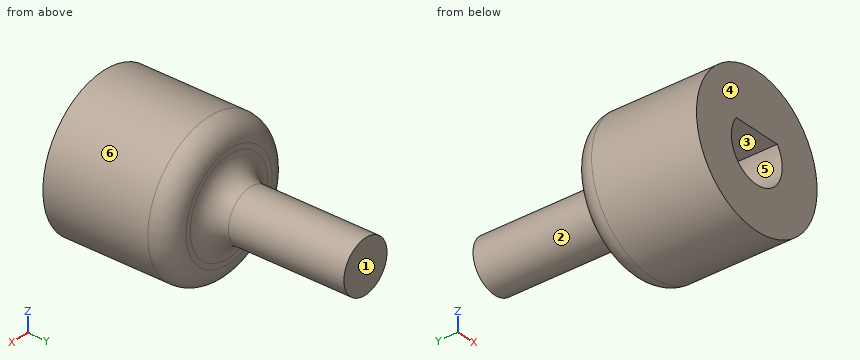
from build123d import *

# Parameters (mm, degrees)
SKETCH1_R           = 12.5
SKETCH1_R_2         = 2
BOSS_EXTRUDE1_DEPTH = 5
SKETCH2_R           = 2.5
BOSS_EXTRUDE2_DEPTH = 15
SKETCH3_R           = 5
CUT_EXTRUDE1_DEPTH  = 2
SKETCH4_R           = 12.5
CUT_EXTRUDE2_DEPTH  = 24.184046239
SKETCH5_R           = 7
SKETCH5_R_2         = 2.95
BOSS_EXTRUDE3_DEPTH = 10
SKETCH5_3_R         = 7
SKETCH5_3_R_2       = 2.95
BOSS_EXTRUDE4_DEPTH = 2
FILLET1_R           = 2
FILLET2_R           = 2


with BuildPart() as part:
    # Sketch1 → Boss-Extrude1 (new body)
    with BuildSketch(Plane(origin=(0, 0, 0), x_dir=(1, 0, 0), z_dir=(0, 1, 0))):
        with Locations(Location((0, 0, 0), (0, 0, 270))):
            Circle(SKETCH1_R)
        with Locations(Location((-7.5, 0, 0), (0, 0, 270))):
            Circle(SKETCH1_R_2, mode=Mode.SUBTRACT)
        with Locations(Location((0, 7.5, 0), (0, 0, 270))):
            Circle(SKETCH1_R_2, mode=Mode.SUBTRACT)
        with Locations(Location((7.5, 0, 0), (0, 0, 270))):
            Circle(SKETCH1_R_2, mode=Mode.SUBTRACT)
        with Locations(Location((0, -7.5, 0), (0, 0, 270))):
            Circle(SKETCH1_R_2, mode=Mode.SUBTRACT)
    extrude(amount=BOSS_EXTRUDE1_DEPTH)

    # Sketch2 → Boss-Extrude2 (add)
    with BuildSketch(Plane(origin=(0, 5, 0), x_dir=(1, 0, 0), z_dir=(0, 1, 0))):
        with Locations(Location((0, 0, 0), (0, 0, 270))):
            Circle(SKETCH2_R)
    extrude(amount=BOSS_EXTRUDE2_DEPTH)

    # Sketch3 → Cut-Extrude1 (cut)
    with BuildSketch(Plane.XZ):
        with Locations(Location((0, 0, 0), (0, 0, 270))):
            Circle(SKETCH3_R)
    extrude(amount=-CUT_EXTRUDE1_DEPTH, mode=Mode.SUBTRACT)

    # Sketch4 → Cut-Extrude2 (cut, through all)
    with BuildSketch(Plane(origin=(0, 5, 0), x_dir=(1, 0, 0), z_dir=(0, 1, 0))):
        Circle(SKETCH4_R)
    extrude(amount=-CUT_EXTRUDE2_DEPTH, mode=Mode.SUBTRACT)

    # Sketch5 → Boss-Extrude3 (add)
    with BuildSketch(Plane.XZ.offset(-5)):
        with Locations(Location((0, 0, 0), (0, 0, 270))):
            Circle(SKETCH5_R)
        Circle(SKETCH5_R_2, mode=Mode.SUBTRACT)
        with BuildLine():
            Line((-1.785357107, 1.75), (0, 1.75))
            Line((0, 1.75), (1.785357107, 1.75))
            ThreePointArc((1.785357107, 1.75), (0, 2.5), (-1.785357107, 1.75))
        make_face()
        with BuildLine():
            ThreePointArc((2.374868417, 1.75), (0, 2.95), (-2.374868417, 1.75))
            Line((-2.374868417, 1.75), (-1.785357107, 1.75))
            ThreePointArc((-1.785357107, 1.75), (0, 2.5), (1.785357107, 1.75))
            Line((1.785357107, 1.75), (2.374868417, 1.75))
        make_face()
    extrude(amount=BOSS_EXTRUDE3_DEPTH)

    # Sketch5_3 → Boss-Extrude4 (add)
    with BuildSketch(Plane.XZ.offset(-5)):
        with Locations(Location((0, 0, 0), (0, 0, 270))):
            Circle(SKETCH5_3_R)
        Circle(SKETCH5_3_R_2, mode=Mode.SUBTRACT)
        with BuildLine():
            Line((-1.785357107, 1.75), (0, 1.75))
            Line((0, 1.75), (1.785357107, 1.75))
            ThreePointArc((1.785357107, 1.75), (0, 2.5), (-1.785357107, 1.75))
        make_face()
        with BuildLine():
            ThreePointArc((2.374868417, 1.75), (0, 2.95), (-2.374868417, 1.75))
            Line((-2.374868417, 1.75), (-1.785357107, 1.75))
            ThreePointArc((-1.785357107, 1.75), (0, 2.5), (1.785357107, 1.75))
            Line((1.785357107, 1.75), (2.374868417, 1.75))
        make_face()
        with BuildLine():
            ThreePointArc((-2.374868417, 1.75), (-2.632964109, -1.33041347), (0, -2.95))
            Line((0, -2.95), (0, -2.5))
            ThreePointArc((0, -2.5), (-2.304886114, -0.968245837), (-1.785357107, 1.75))
            Line((-1.785357107, 1.75), (-2.374868417, 1.75))
        make_face()
        with BuildLine():
            Line((0, -2.5), (0, -2.95))
            ThreePointArc((0, -2.95), (2.085965005, -2.085965005), (2.95, 0))
            ThreePointArc((2.95, 0), (2.802531162, 0.92104239), (2.374868417, 1.75))
            Line((2.374868417, 1.75), (1.785357107, 1.75))
            ThreePointArc((1.785357107, 1.75), (2.314453798, 0.945147404), (2.5, 0))
            ThreePointArc((2.5, 0), (1.767766953, -1.767766953), (0, -2.5))
        make_face()
        with BuildLine():
            ThreePointArc((-1.785357107, 1.75), (-2.304886114, -0.968245837), (0, -2.5))
            Line((0, -2.5), (0, 1.75))
            Line((0, 1.75), (-1.785357107, 1.75))
        make_face()
        with BuildLine():
            Line((0, 1.75), (0, -2.5))
            ThreePointArc((0, -2.5), (1.767766953, -1.767766953), (2.5, 0))
            ThreePointArc((2.5, 0), (2.314453798, 0.945147404), (1.785357107, 1.75))
            Line((1.785357107, 1.75), (0, 1.75))
        make_face()
    extrude(amount=-BOSS_EXTRUDE4_DEPTH)

    # Fillet1
    fillet1_edges = [part.edges().sort_by_distance(p)[0] for p in [
        (0, 7, -2.5),
    ]]
    fillet(fillet1_edges, radius=FILLET1_R)

    # Fillet2
    fillet2_edges = [part.edges().sort_by_distance(p)[0] for p in [
        (0, 7, 7),
    ]]
    fillet(fillet2_edges, radius=FILLET2_R)


solid = part.part
Part model, mm, in its own coordinate system. Face numbers are marked on the shaded views. A direction names the side the tool comes from. Coordinates: 2 decimals unless noted, no trailing zeros. Write each loop counter-clockwise with the first axis right and the second up, starting at its lowest first coordinate (ties: lowest second). Pieces come first, ordered by that corner, then holes. Notation, with made-up numbers: (60.25, 29.5) - (70.25, 29.5) arc R30 ccw to (70.25, 61.5) - close; hole circle Ø4 at (44.25, 89.5). An arc over 180 degrees is marked (long way). Put each result on its own line as item: value.
1. 3-axis set-ups, long thin cutter, end or side, ignore diameter. For the marked faces 1 and 2: which of +Z, -Z, +X, -X, +Y, -Y reach the whole face in a straight line?
Final values:
face 1: +Z, -Z, +X, -X, +Y
face 2: +Y
2. Probe line 1 along X through (y, z) = (1.75, 0); line 2 along X through (y, z) = (-1, 1); line 3 along Z through (x, y) = (2.5, 2.75). List the from-to ranges inside material, lowest first. Write a range as [from, to].
Final values:
line 1: x = [-7, -2.95], [2.95, 7]
line 2: x = [-6.93, -2.78], [2.78, 6.93]
line 3: z = [-6.54, -1.57], [1.57, 6.54]
3. Band-saw the part on A-A (x = 0). Write the cut outline in (y, z).
Final values:
outline: (-5, -7) - (5, -7) arc R2 ccw to (7, -5) - (7, -4.5) arc R2 cw to (9, -2.5) - (20, -2.5) - (20, 2.5) - (9, 2.5) arc R2 cw to (7, 4.5) - (7, 5) arc R2 ccw to (5, 7) - (-5, 7) - (-5, 1.75) - (5, 1.75) - (5, -2.95) - (-5, -2.95) - close
4. Band-saw the part on B-B (z = 0). Write the cut outline in (x, y).
Final values:
outline: (-7, -5) - (-2.95, -5) - (-2.95, 5) - (2.95, 5) - (2.95, -5) - (7, -5) - (7, 5) arc R2 ccw to (5, 7) - (4.5, 7) arc R2 cw to (2.5, 9) - (2.5, 20) - (-2.5, 20) - (-2.5, 9) arc R2 cw to (-4.5, 7) - (-5, 7) arc R2 ccw to (-7, 5) - close
5. Band-saw the part on C-C (y = -1.25). Write the cut outline in (x, z).
Final values:
outline: circle Ø14 at (0, 0); hole (-2.37, 1.75) arc R2.95 ccw (long way) to (2.37, 1.75) - close
6. Band-saw the part on D-D (y = 17). Write the cut outline in (x, z).
Final values:
outline: circle Ø5 at (0, 0)
7. Two-plate mould, pull along Z, no slides. Class the marked faces 3, 4, 5 and 6: +Z half, -Z half, draft (parallel to the pull), parting line (faces both ways), or undercut.
Final values:
face 3: undercut
face 4: draft
face 5: undercut
face 6: parting line
8. Flat gauge pins, fed straight in: pin 1 Ø6 at (x, y) = (-4, 11.5) entering from +Z; pin 2 Ø1.5 at (x, z) = (-3.5, 4.5) entering from +Y; pin 3 Ø6 at (x, z) = (-3.5, -5) entering from +Y. Where does each tip first touch, or does it go through?
Final values:
pin 1: stops at z = 2.29
pin 2: stops at y = 7
pin 3: stops at y = 7.57
